Autodesk Inventor part; units mm, degrees
ref_plane "YZ Plane" through (0, 0, 0) normal (1, 0, 0) x (0, 1, 0)
ref_plane "XZ Plane" through (0, 0, 0) normal (0, 1, 0) x (-1, 0, 0)
ref_plane "XY Plane" through (0, 0, 0) normal (0, 0, 1) x (1, 0, 0)
sketch "Sketch1" plane through (0, 0, 0) normal (0, 1, 0) x (-1, 0, 0)
  line L0 (0, 0) -> (2.5, 0)
  line L1 (2.5, 0) -> (2.5, 4)
  line L2 (2.5, 4) -> (4, 4)
  line L3 (4, 4) -> (4, 5)
  line L4 (4, 5) -> (0, 5)
  line L5 (0, 5) -> (0, 0)
  dimension "d0" = 2.5
  dimension "d1" = 4
  dimension "d2" = 1.5
revolve "Revolution1" add sketch "Sketch1" angle 360 about axis through (0, 0, 5) along (0, 0, -1)
thread "Thread1"
sketch "Sketch2" plane through (0, 0, 5) normal (0, 0, 1) x (1, 0, 0)
  line L0 (5, 2.8868) -> (5, -2.8868)
  line L1 (5, -2.8868) -> (0, -5.7735)
  line L2 (0, -5.7735) -> (-5, -2.8868)
  line L3 (-5, -2.8868) -> (-5, 2.8868)
  line L4 (-5, 2.8868) -> (0, 5.7735)
  line L5 (0, 5.7735) -> (5, 2.8868)
  point P0 (0, 0)
  point P1 (0, 0)
  dimension "d9" = 10
extrude "Extrusion1" add sketch "Sketch2" along normal blind 7.5
sketch "Sketch3" plane through (0, 0, 12.5) normal (0, 0, 1) x (1, 0, 0)
  circle A0 centre (0, 0) radius 5
  dimension "d12" = 10
extrude "Extrusion2" add sketch "Sketch3" along normal blind 2.5
fillet "Fillet1" radius 1.5 1 edges at (-5, 0, 15)
sketch "Sketch4" plane through (0, 0, 15) normal (0, 0, 1) x (1, 0, 0)
  circle A0 centre (0, 0) radius 2.5
  dimension "d16" = 5
extrude "Extrusion3" add sketch "Sketch4" along normal blind 1.5
sketch "Sketch5" plane through (0, 0, 16.5) normal (0, 0, 1) x (1, 0, 0)
  circle A0 centre (0, 0) radius 5.5
  dimension "d19" = 11
extrude "Extrusion4" add sketch "Sketch5" along normal blind 1
sketch "Sketch6" plane through (0, 0, 17.5) normal (0, 0, 1) x (1, 0, 0)
  circle A0 centre (0, 0) radius 2.5
hole "Hole1" at (0, 0, 17.5) direction (0, 0, -1) diameter 4 end through all
fillet "Fillet2" radius 0.1 2 edges at (-5.5, 0, 17.5) (-5.5, 0, 16.5)
fillet "Fillet3" radius 0.2 6 edges at (0, -5.7735, 8.75) (5, -2.8868, 8.75) (5, 2.8868, 8.75) (0, 5.7735, 8.75) (-5, 2.8868, 8.75) (-5, -2.8868, 8.75)
sketch "Sketch7" plane through (0, 0, 15) normal (0, 0, 1) x (1, 0, 0)
  circle A0 centre (0, 0) radius 3.5
extrude "Extrusion5" add sketch "Sketch7" along normal blind 0.75
properties part number "Bowden"
Could you check a few things on this model? Use its own coordinates, in mm. A direction names the side the tool comes from. Round coordinates to 2 decimals unless told otherwise and drop trailing zeros. Loops run counter-clockwise (first coordinate to the right, second up) from the corner with the lowest first, then second, coordinate; pieces in that order, holes last. Notation, with made-up numbers: (75.25, 12.5) - (105.25, 12.5) arc R23 ccw to (105.25, 25.5) - close; hole circle Ø7 at (-10.75, 80.5). An arc over 180 degrees is marked (long way). Answer as CSV lines item,"result".
1. I want a section at B-B on z = 4.75. List the corners of the cut face in (x, y) for me, then the cut area to 3 significant figures.
Filled in:
outline,"circle Ø8 at (0, 0); hole circle Ø4 at (0, 0)"
area,"37.7 mm^2"
2. We'd pull the mould along X, two halves only. Please class faces 4 (the face through (2, 0, 7)), 5 (the face through (2.534, -4.311, 8.698)), 6 (the face through (-5, 0, 9)): +X half, -X half, draft (parallel to the pull), parting line (faces both ways), or undercut.
Filled in:
face 4,"undercut"
face 5,"+X half"
face 6,"-X half"
3. For pin 1 Ø1.5 at (y, z) = (1.5, 6) entering from +X; pin 2 Ø3 at (x, y) = (0, 0) entering from +Z; pin 3 Ø5 at (y, z) = (-1, 11) entering from -X, each with a flat end and sliding along its axis, tell me the tip position at first contact or that it passes through.
Filled in:
pin 1,"stops at x = 5"
pin 2,"stops at z = 15.75"
pin 3,"stops at x = -5"
4. Please list where these lines run through material, in increasing order: line 1 along Z through (x, y) = (2.5, 2.5); line 2 along X through (y, z) = (0, 16.2); line 3 along Z through (x, y) = (-2.25, -1.5). Write a range as [from, to].
Filled in:
line 1,"z = [4, 15], [16.5, 17.5]"
line 2,"x = [-2.5, -2], [2, 2.5]"
line 3,"z = [4, 15.75], [16.5, 17.5]"
5. I want a section at A-A on z = 8. List the corners of the cut face in (x, y) for me, then the cut area to 3 significant figures.
Filled in:
outline,"(-5, -2.77) arc R0.2 ccw to (-4.9, -2.94) - (-0.1, -5.72) arc R0.2 ccw to (0.1, -5.72) - (4.9, -2.94) arc R0.2 ccw to (5, -2.77) - (5, 2.77) arc R0.2 ccw to (4.9, 2.94) - (0.1, 5.72) arc R0.2 ccw to (-0.1, 5.72) - (-4.9, 2.94) arc R0.2 ccw to (-5, 2.77) - close; hole circle Ø4 at (0, 0)"
area,"74.0 mm^2"
6. On a 3-axis mill with a long thin cutter (end or side, diameter ignored), from which of +Z, -Z, +X, -X, +Y, -Y can I reach the whole of each face in a straight line? I mean faces 1 (the face through (-1.08, 4.88, 12.99)), 2 (the face through (2.466, 4.35, 8.698)), 3 (the face through (-2.534, 4.311, 8.698)). Say none if no direction works.
Filled in:
face 1,"none"
face 2,"-Z, +X, +Y"
face 3,"-Z, -X, +Y"
